Check sheet for the drawn part. Datum: minimum x, y, z corner. Units: mm. Round coordinates to 2 decimals unless told otherwise and drop trailing zeros. Write each loop counter-clockwise with the first axis right and the second up, starting at its lowest first coordinate (ties: lowest second). Pieces come first, ordered by that corner, then holes.
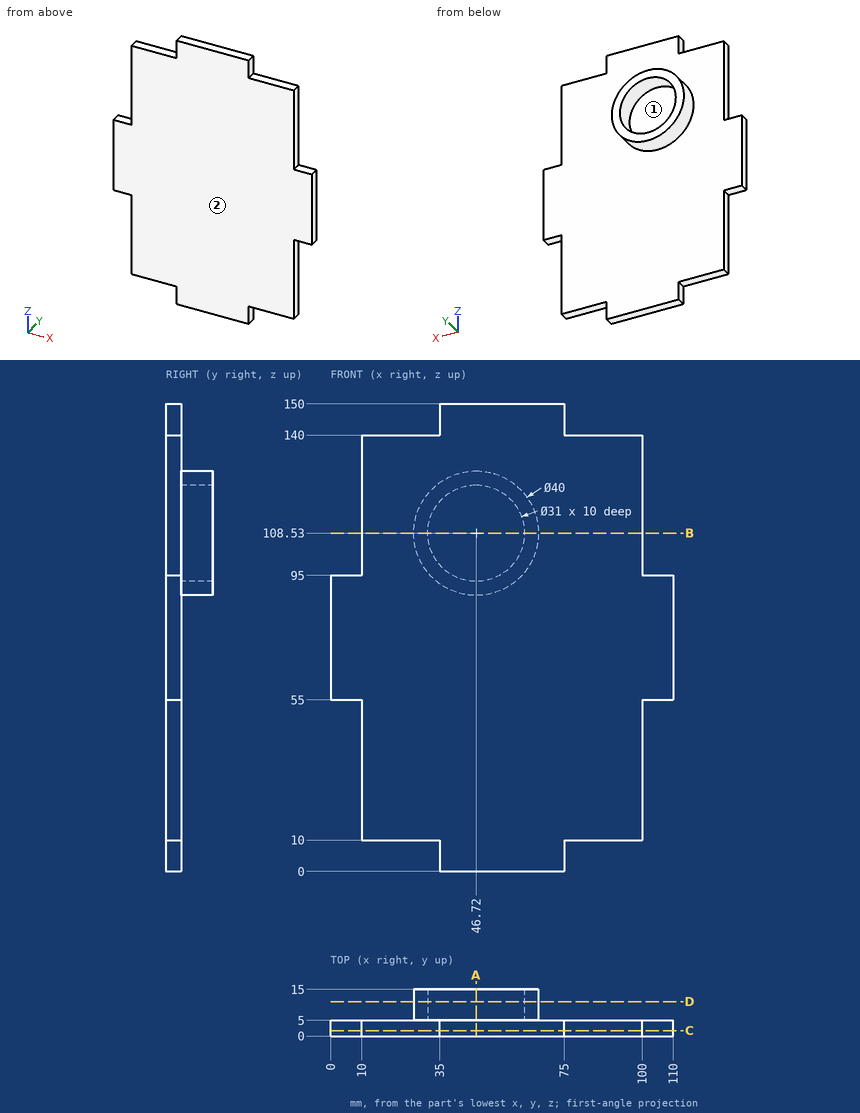
Q1. Sectioned sample at D-D (y = 11). Enter the section's corners in (x, z), plus the area to 3 significant figures.
Recorded:
outline: circle Ø40 at (46.72, 108.53); hole circle Ø31 at (46.72, 108.53)
area: 502 mm2
Q2. Sectioned sample at C-C (y = 1.75). Enter the section's corners in (x, z).
Recorded:
outline: (0, 55) - (10, 55) - (10, 10) - (35, 10) - (35, 0) - (75, 0) - (75, 10) - (100, 10) - (100, 55) - (110, 55) - (110, 95) - (100, 95) - (100, 140) - (75, 140) - (75, 150) - (35, 150) - (35, 140) - (10, 140) - (10, 95) - (0, 95) - close
Q3. Sectioned sample at B-B (z = 108.53). Enter the section's corners in (x, y).
Recorded:
outline: (10, 0) - (100, 0) - (100, 5) - (66.72, 5) - (66.72, 15) - (62.22, 15) - (62.22, 5) - (31.22, 5) - (31.22, 15) - (26.72, 15) - (26.72, 5) - (10, 5) - close
Q4. Release check for a two-part mould opening along X. For the marked faces 1 and 2 record: released by +X, released by -X, zero draft, split by the parting line, or undercut.
Recorded:
face 1: undercut
face 2: zero draft
Q5. Depth check by flat-ended pin: P1, Ø5.5, axis at y = 2, z = 7, coming from the -X side; P2, Ø1.5, axis at y = 2, z = 112.5, coming from the +X side; P3, Ø2, axis at x = 55, z = 83.5, coming from the +Y side. Enter the tip coordinate at first touch or a pass-through.
Recorded:
P1: stops at x = 35
P2: stops at x = 100
P3: stops at y = 5
Q6. Sectioned sample at A-A (x = 46.72). Enter the section's corners in (y, z), plus the area to 3 significant figures.
Recorded:
outline: (0, 0) - (5, 0) - (5, 88.53) - (15, 88.53) - (15, 93.03) - (5, 93.03) - (5, 124.03) - (15, 124.03) - (15, 128.53) - (5, 128.53) - (5, 150) - (0, 150) - close
area: 840 mm2
Q7. Material ranges on line 1 along X through (y, z) = (3.25, 135.5); line 2 along X through (y, z) = (10.5, 108.53); line 3 along Y through (x, z) = (11.5, 59), recorded low to high.
Recorded:
line 1: x = 10 to 100
line 2: x = 26.72 to 31.22, 62.22 to 66.72
line 3: y = 0 to 5
